Geometry: final body of the model. Coordinates: model frame, mm. Round coordinates to 2 decimals unless told otherwise and drop trailing zeros. Order: outer loops, then holes, each group sorted by start corner. A loop starts at its lowest first (then second) coordinate and runs counter-clockwise, first axis right, second up. Notation, with made-up numbers: M -32.5,58.5 L -3.5,58.5 A31 ccw -3.5,92.5 Z; hole C 45,14.5 d8. An arc over 180 degrees is marked long. Put each result on its own line as item: value. Start each with the question number.
1) Material intervals for probe 1 along Z at (x, y) = (1, 2.4); probe 2 along Z at (x, y) = (-4.5, 2.2); probe 3 along Y at (x, z) = (3.5, -1), sorted ascending. Write a range as [from, to].
2) First-contact query: P1, Ø0.5, axis at x = 2, y = 2.5, coming from the +Z side; P2, Ø2.5, axis at x = -0.5, z = -4.5, coming from the +Y side; P3, Ø0.5, axis at x = -1.5, y = 2.5, coming from the -Z side. Flat tips, straight axial feed; report the tip coordinate or a pass-through.
3) Section B-B, the plane y = 0.75. Return loops of the section in (x, z).
4) Section D-D, the plane z = -17. Return loops of the section in (x, y).
5) Draft query along X for faces 1 (the flat face through (0, 0, 0)), 2 (the flat face through (0, 2, -4)), 3 (the cylindrical face through (4.336, 1.282, 19.524)). Return one class per face: pulls with the +X half, pulls with the -X half, needs draft (parallel to the pull), parting line crosses it, or undercut.
6) Section A-A, the plane x = -1.5. Return loops of the section in (y, z).
7) Section C-C, the plane x = -6. Return loops of the section in (y, z), then the cut area to 3 significant figures.
Autodesk Inventor part; units mm, degrees
ref_plane "YZ Plane" through (0, 0, 0) normal (1, 0, 0) x (0, 1, 0)
ref_plane "XZ Plane" through (0, 0, 0) normal (0, 1, 0) x (-1, 0, 0)
ref_plane "XY Plane" through (0, 0, 0) normal (0, 0, 1) x (1, 0, 0)
sketch "Sketch1" plane through (0, 0, 0) normal (0, 1, 0) x (-1, 0, 0)
  circle A0 centre (0, 0) radius 20
  dimension "d0" = 40
extrude "Extrusion1" add sketch "Sketch1" along normal blind 2.6
sketch "Sketch2" plane through (0, 2.6, 0) normal (0, 1, 0) x (1, 0, 0)
  line L0 (-10, -10) -> (-10, 10)
  line L1 (-10, 10) -> (10, 10)
  line L2 (10, 10) -> (10, -10)
  line L3 (10, -10) -> (-10, -10)
  line L4 (-10, -10) -> (10, 10) construction
  line L5 (-10, 10) -> (10, -10) construction
  point P0 (0, 0)
  dimension "d3" = 20
  dimension "d4" = 20
extrude "Extrusion2" cut sketch "Sketch2" against normal blind 0.6
sketch "Sketch3" plane through (0, 2, 0) normal (0, 1, 0) x (1, 0, 0)
  line L0 (-6.6897, 8.3364) -> (6.7624, 8.3364) construction
  line L1 (6.7624, 8.3364) -> (6.7624, -8.2636) construction
  line L2 (6.7624, -8.2636) -> (-6.6897, -8.2636) construction
  line L3 (-6.6897, -8.2636) -> (-6.6897, 8.3364) construction
  spline S0 degree 2 poles (6.2513, -3.1653) (6.2513, -4.4029) (5.3096, -6.2996) (4.5294, -6.9184) knots 0 0 0 1 2 2 2
  spline S1 degree 2 poles (4.5294, -6.9184) (3.5877, -7.6448) (1.4488, -8.2636) (-0.2461, -8.2636) knots 0 0 0 1 2 2 2
  line L4 (-0.2461, -8.2636) -> (-5.0082, -8.2636)
  line L5 (-5.0082, -8.2636) -> (-5.0082, 8.3364)
  line L6 (-5.0082, 8.3364) -> (-0.6094, 8.3364)
  spline S2 degree 2 poles (-0.6094, 8.3364) (1.1663, 8.3364) (2.942, 8.1077) (3.7492, 7.6637) knots 0 0 0 1 2 2 2
  spline S3 degree 2 poles (3.7492, 7.6637) (4.6505, 7.1929) (5.471, 5.6459) (5.471, 4.5966) knots 0 0 0 1 2 2 2
  spline S4 degree 2 poles (5.471, 4.5966) (5.471, 3.4263) (4.2334, 1.5699) (3.1438, 1.0453) knots 0 0 0 1 2 2 2
  line L7 (3.1438, 1.0453) -> (3.1438, 0.9646)
  spline S5 degree 2 poles (3.1438, 0.9646) (4.6235, 0.561) (6.2513, -1.5779) (6.2513, -3.1653) knots 0 0 0 1 2 2 2
  spline S6 degree 2 poles (3.9509, -3.2594) (3.9509, -2.3178) (3.4129, -1.1071) (2.6057, -0.6766) knots 0 0 0 1 2 2 2
  spline S7 degree 2 poles (2.6057, -0.6766) (2.0811, -0.4076) (0.8435, -0.2461) (-0.3, -0.2461) knots 0 0 0 1 2 2 2
  line L8 (-0.3, -0.2461) -> (-2.8021, -0.2461)
  line L9 (-2.8021, -0.2461) -> (-2.8021, -6.3803)
  line L10 (-2.8021, -6.3803) -> (-1.0129, -6.3803)
  spline S8 degree 2 poles (-1.0129, -6.3803) (0.4399, -6.3803) (2.108, -6.1113) (2.7537, -5.6808) knots 0 0 0 1 2 2 2
  spline S9 degree 2 poles (2.7537, -5.6808) (3.3725, -5.2369) (3.9509, -4.1338) (3.9509, -3.2594) knots 0 0 0 1 2 2 2
  spline S10 degree 2 poles (3.1707, 4.2872) (3.1707, 4.8791) (2.7671, 5.767) (2.3232, 6.0226) knots 0 0 0 1 2 2 2
  spline S11 degree 2 poles (2.3232, 6.0226) (1.7851, 6.3185) (0.4803, 6.453) (-0.6901, 6.453) knots 0 0 0 1 2 2 2
  line L11 (-0.6901, 6.453) -> (-2.8021, 6.453)
  line L12 (-2.8021, 6.453) -> (-2.8021, 1.5968)
  line L13 (-2.8021, 1.5968) -> (-0.3, 1.5968)
  spline S12 degree 2 poles (-0.3, 1.5968) (0.7359, 1.5968) (1.7179, 1.812) (2.2425, 2.1483) knots 0 0 0 1 2 2 2
  spline S13 degree 2 poles (2.2425, 2.1483) (2.7537, 2.4712) (3.1707, 3.507) (3.1707, 4.2872) knots 0 0 0 1 2 2 2
  point P0 (0, 0)
extrude "Extrusion3" add sketch "Sketch3" along normal blind 0.6
properties part number "TopMarkerPreset"
Result sheet:
1. probe 1: z = [-19.97, -10], [-8.31, -6.4], [-1.66, 0.28], [6.28, 8.21], [10, 19.97]
1. probe 2: z = [-19.49, -10], [-8.34, 8.26], [10, 19.49]
1. probe 3: y = [0, 2]
2. P1: stops at z = 19.92
2. P2: stops at y = 2
2. P3: stops at z = -19.96
3. outline: C 0,0 d40
4. outline: M -10.54,0 L 10.54,0 L 10.54,2.6 L -10.54,2.6 Z
5. face 1: needs draft
5. face 2: undercut
5. face 3: parting line crosses it
6. outline: M 0,-19.94 L 2.6,-19.94 L 2.6,-10 L 2,-10 L 2,-8.34 L 2.6,-8.34 L 2.6,-6.45 L 2,-6.45 L 2,-1.6 L 2.6,-1.6 L 2.6,0.25 L 2,0.25 L 2,6.38 L 2.6,6.38 L 2.6,8.26 L 2,8.26 L 2,10 L 2.6,10 L 2.6,19.94 L 0,19.94 Z
7. outline: M 0,-19.08 L 2.6,-19.08 L 2.6,-10 L 2,-10 L 2,10 L 2.6,10 L 2.6,19.08 L 0,19.08 Z
7. area: 87.2 mm2
